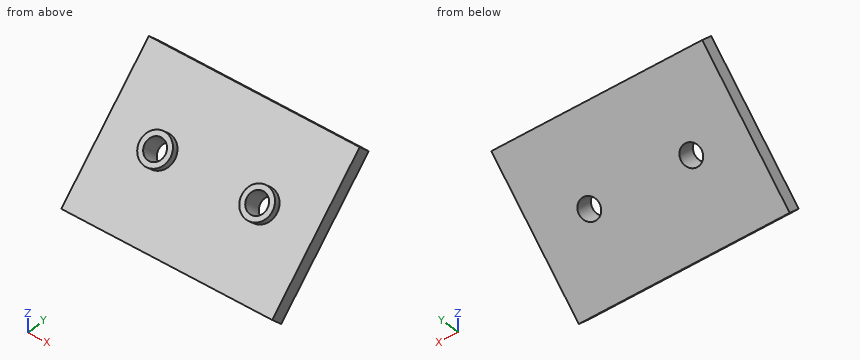
```python
from build123d import *

# Parameters (mm, degrees)
SKETCH1_W                = 41
SKETCH1_H                = 29
BOSS_EXTRUDE1_DEPTH      = 3
SKETCH11_R               = 3
BOSS_EXTRUDE2_DEPTH      = 1.5
F_4_0_4_DIAMETER_HOLE1_D = 4
BODY_MOVE_COPY9_ANGLE    = 45


with BuildPart() as part:
    # Sketch1 → Boss-Extrude1 (new body)
    with BuildSketch(Plane.XY):
        Rectangle(SKETCH1_W, SKETCH1_H)
    extrude(amount=BOSS_EXTRUDE1_DEPTH)


with BuildPart() as part_1:
    # Body-Move/Copy1: moved
    add(part.part.moved(Location((0.5, 0.5, 0))))

    # Sketch11 → Boss-Extrude2 (add)
    with BuildSketch(Plane.XY.offset(3)):
        with Locations((-9.387244392, 0.5)):
            Circle(SKETCH11_R)
        with Locations((10.452938647, 0.5)):
            Circle(SKETCH11_R)
    extrude(amount=BOSS_EXTRUDE2_DEPTH)

    # Ø4.0 (4) Diameter Hole1 (through all)
    with Locations(Plane.XY.offset(4.5)):
        with Locations((-9.387244392, 0.5), (10.452938647, 0.5)):
            Hole(F_4_0_4_DIAMETER_HOLE1_D / 2)


with BuildPart() as part_2:
    # Body-Move/Copy8: moved
    add(part_1.part.moved(Location((27.795693281, 0, 0))))


with BuildPart() as part_3:
    # Body-Move/Copy9: moved
    add(part_2.part.rotate(Axis((0, 0.5, 2.25), (1, 0, 0)), BODY_MOVE_COPY9_ANGLE))


solid = part_3.part
```
Here's how the part is built. I have some questions about the finished solid (model axes, mm). Coordinates: 2 decimals unless noted, no trailing zeros. Write each loop counter-clockwise with the first axis right and the second up, starting at its lowest first coordinate (ties: lowest second). Pieces come first, ordered by that corner, then holes. Notation, with made-up numbers: M 76,-2 L 124,-2 A18 cw 124,28 Z; hole C 1.5,-23.5 d8. An arc over 180 degrees is marked long. Answer as CSV lines item,"result". Start each with the question number.
Q1. Will these pins go through, and if not, where does the flat tip stop? pin 1 Ø3 at (x, y) = (39, 6) entering from +Z; pin 2 Ø3 at (x, y) = (28, 1) entering from +Z; pin 3 Ø1.5 at (x, z) = (23, -2) entering from -Y.
Q2. I need wall thicknesses on probe 1 along Z at (x, y) = (26, -7.5); probe 2 along Z at (x, y) = (28.5, -6); probe 3 along Y at (x, z) = (35, -1). Which ranges of each line are inside material? Lowest first, please. Write a range as [from, to].
Q3. Suppose I cut it at A-A, the plane z = 6.5. List the corners of the cut face in (x, y) for me, then the cut area to 3 significant figures.
Q4. Suppose I cut it at B-B, the plane x = 43.5. List the corners of the cut face in (y, z) for me.
Entries:
1,pin 1,"stops at z = 10.31"
1,pin 2,"stops at z = 5.31"
1,pin 3,"stops at y = -5.56"
2,probe 1,"z = [-8.93, -4.69]"
2,probe 2,"z = [-7.43, -3.19]"
2,probe 3,"y = [-3.81, 0.43]"
3,outline,"M 7.8,3.69 L 48.8,3.69 L 48.8,7.93 L 7.8,7.93 Z"
3,area,"174 mm²"
4,outline,"M -10.28,-7.47 L -8.16,-9.59 L 12.34,10.91 L 10.22,13.03 Z"
